Here's how the part is built. I have some questions about the finished solid (model axes, mm). A direction names the side the tool comes from. Round coordinates to 2 decimals unless told otherwise and drop trailing zeros. Order: outer loops, then holes, each group sorted by start corner. A loop starts at its lowest first (then second) coordinate and runs counter-clockwise, first axis right, second up. Notation, with made-up numbers: (58.25, -33.75) -> (106.25, -33.75) arc R12 ccw to (106.25, -11.75) -> close; hole circle Ø4 at (85, 88). An arc over 180 degrees is marked (long way). Answer in a Markdown table with one row per item.
```python
from build123d import *

# Parameters (mm, degrees)
CROQUIS2_W              = 1
CROQUIS2_H              = 350
SALIENTE_EXTRUIR2_DEPTH = 25
CROQUIS5_R              = 1.5
CORTAR_EXTRUIR2_DEPTH   = 1
CROQUIS1_R              = 1.5
SALIENTE_EXTRUIR3_DEPTH = 1


with BuildPart() as part:
    # Croquis2 → Saliente-Extruir2 (new body)
    with BuildSketch(Plane.XY):
        with Locations((-54.941785307, -113.819624774)):
            Rectangle(CROQUIS2_W, CROQUIS2_H)
    extrude(amount=SALIENTE_EXTRUIR2_DEPTH)

    # Croquis5 → Cortar-Extruir2 (cut)
    with BuildSketch(Plane(origin=(-54.441785307, 0, 0), x_dir=(0, 0, -1), z_dir=(1, 0, 0))):
        with Locations((-20, 43.180375226)):
            Circle(CROQUIS5_R)
        with Locations((-20, -270.819624774)):
            Circle(CROQUIS5_R)
    extrude(amount=-CORTAR_EXTRUIR2_DEPTH, mode=Mode.SUBTRACT)

    # Croquis1 → Saliente-Extruir3 (add)
    with BuildSketch(Plane.XY):
        Polygon((-55.441785307, 61.180375226), (-79.441785307, 37.180375226), (-79.441785307, -264.819624774), (-55.441785307, -288.819624774), align=None)
        with Locations((-74.441785307, 1.180375226)):
            Circle(CROQUIS1_R, mode=Mode.SUBTRACT)
        with Locations((-74.441785307, -228.819624774)):
            Circle(CROQUIS1_R, mode=Mode.SUBTRACT)
    extrude(amount=SALIENTE_EXTRUIR3_DEPTH)


solid = part.part
```
1. Suppose I cut it at C-C on x = -67.75. Write out the boundary of the cut face in (y, z).
Numbers:
| item | result |
|---|---|
| outline | (-276.51, 0) -> (48.87, 0) -> (48.87, 1) -> (-276.51, 1) -> close |
2. Please list where these lines run through material, in increasing order: line 1 along Y through (x, z) = (-55.15, 20); line 2 along Z through (x, y) = (-57.5, -14.5); line 3 along X through (y, z) = (-117.5, 20).
Numbers:
| item | result |
|---|---|
| line 1 | y = -288.82 to -272.32, -269.32 to 41.68, 44.68 to 61.18 |
| line 2 | z = 0 to 1 |
| line 3 | x = -55.44 to -54.44 |
3. For pin 1 Ø1.8 at (x, y) = (-74.44, -228.82) entering from -Z; pin 2 Ø4 at (x, y) = (-74.44, 1.18) entering from +Z; pin 3 Ø5 at (y, z) = (43.18, 20) entering from +X; pin 4 Ø12 at (y, z) = (-81.5, 14.5) entering from -X, each with a flat end and sliding along its axis, tell me the tip position at first contact or that it passes through.
Numbers:
| item | result |
|---|---|
| pin 1 | passes through |
| pin 2 | stops at z = 1 |
| pin 3 | stops at x = -54.44 |
| pin 4 | stops at x = -55.44 |
4. Suppose I cut it at A-A on y = -113. Write out the boundary of the cut face in (x, z).
Numbers:
| item | result |
|---|---|
| outline | (-79.44, 0) -> (-54.44, 0) -> (-54.44, 25) -> (-55.44, 25) -> (-55.44, 1) -> (-79.44, 1) -> close |
5. Suppose I cut it at B-B on z = 11. Write out the boundary of the cut face in (x, y), then the cut area to 3 significant figures.
Numbers:
| item | result |
|---|---|
| outline | (-55.44, -288.82) -> (-54.44, -288.82) -> (-54.44, 61.18) -> (-55.44, 61.18) -> close |
| area | 350 mm2 |
6. For faces 1 (the face through (-54.442, -116, 12)), 2 (the face through (-55.442, -116, 13)), which set-ups out of +Z, -Z, +X, -X, +Y, -Y let a thin tool reach every point of the face, with its end or its side?
Numbers:
| item | result |
|---|---|
| face 1 | +Z, -Z, +X, +Y, -Y |
| face 2 | +Z, -X, +Y, -Y |
